For this review, use the dimensioned drawing (mm, ordinates from the lowest corner) and the shaded views. A direction names the side the tool comes from. Give positions to 0.01 mm unless a question says otherwise; leave off trailing zeros. Loops run counter-clockwise (first coordinate to the right, second up) from the corner with the lowest first, then second, coordinate; pieces in that order, holes last. Notation, with made-up numbers: M 77.25,40.25 L 101.25,40.25 A20 ccw 101.25,45.25 Z; hole C -4,-10 d8. An arc over 180 degrees is marked long. Use CSV: the item, a comma, the result in double quotes. Start each with the question number.
1. Take a section at C-C, the plane z = 6.5. Write out the cut boundary in (x, y) (3 decimals).
2. Take a section at D-D, the plane y = 19.5. Write out the cut boundary in (x, z), and give its area (3 significant figures).
3. Insertion check: P1, Ø1.5, axis at x = 26, z = 4, coming from the +Y side; P2, Ø1, axis at x = 13.5, y = 12.5, coming from the +Z side; P3, Ø4, axis at x = 16, z = 12.5, coming from the +Y side; P4, Ø4.5, axis at y = 16, z = 7.5, coming from the -X side (3 decimals). Each pin has a flat end and moves straight along its axis. Give the tip position at first contact, or say it passes through.
4. Tool access review of the marked faces 4 and 5: name each direction out of +Z, -Z, +X, -X, +Y, -Y from which nothing blocks a thin tool from reaching the whole face with its end or side.
5. To check wall thickness, follow line 1 (X direction, y = 16, z = 10.75) (3 decimals); line 2 (Z direction, x = 3, y = 25). State the ranges of each line that lie inside material, in increasing order. Write a range as [from, to].
6. Take a section at A-A, the plane x = 16. Write out the cut boundary in (y, z) (3 decimals).
7. The part is to be moulded in two halves that separate along Z. For the marked faces 1, 2 and 3, say which applies: pulls with the +Z half, pulls with the -Z half, needs draft (parallel to the pull), parting line crosses it, or undercut.
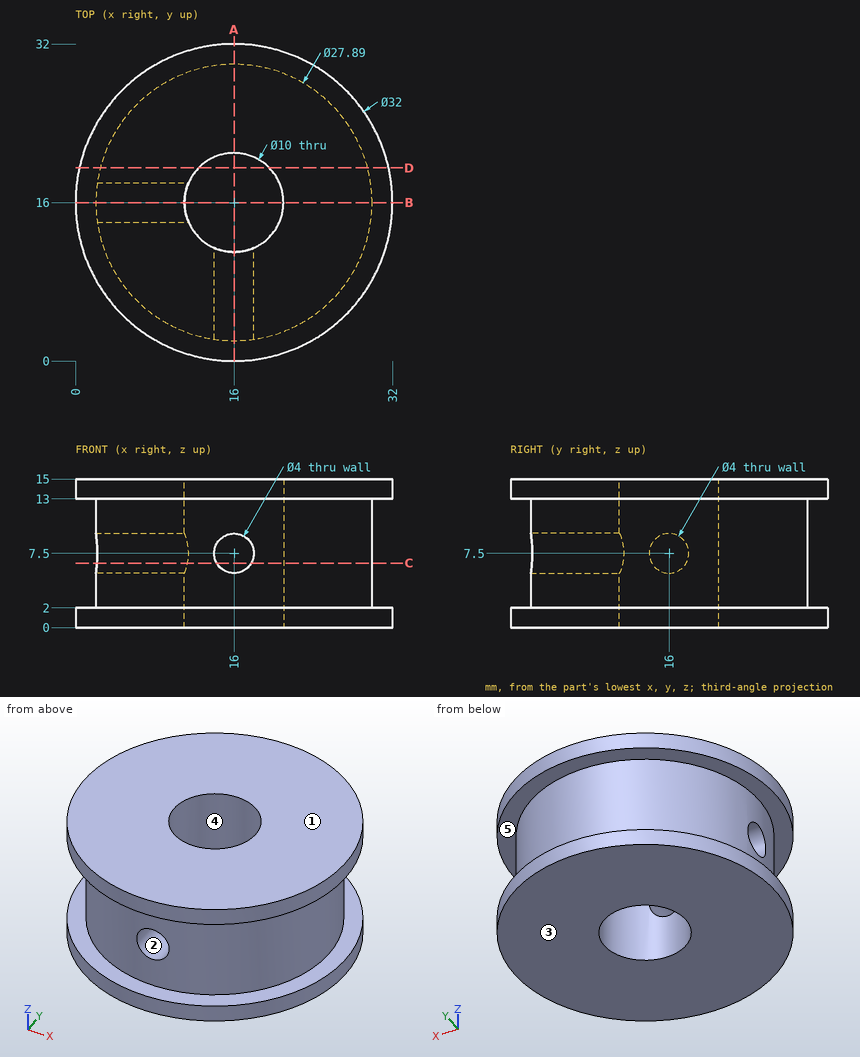
Result set:
1,outline,"M 2.163,14.268 A13.945 ccw 14.268,2.163 L 14.268,11.31 A5 cw 11.31,14.268 Z; M 2.163,17.732 L 11.31,17.732 A5 cw long 17.732,11.31 L 17.732,2.163 A13.945 ccw long Z"
2,outline,"M 0.39,0 L 12.43,0 L 12.43,15 L 0.39,15 L 0.39,13 L 2.5,13 L 2.5,2 L 0.39,2 Z; M 19.57,0 L 31.61,0 L 31.61,2 L 29.5,2 L 29.5,13 L 31.61,13 L 31.61,15 L 19.57,15 Z"
2,area,"315 mm2"
3,P1,"y = 26.44"
3,P2,"through"
3,P3,"y = 32"
3,P4,"x = 2.055"
4,face 4,"+Z, -Z"
4,face 5,"none"
5,line 1,"[2.055, 11], [21, 29.945]"
5,line 2,"[0, 2], [13, 15]"
6,outline,"M 0,0 L 11,0 L 11,5.5 L 2.055,5.5 L 2.055,2 L 0,2 Z; M 0,13 L 2.055,13 L 2.055,9.5 L 11,9.5 L 11,15 L 0,15 Z; M 21,0 L 32,0 L 32,2 L 29.945,2 L 29.945,13 L 32,13 L 32,15 L 21,15 Z"
7,face 1,"pulls with the +Z half"
7,face 2,"undercut"
7,face 3,"pulls with the -Z half"
